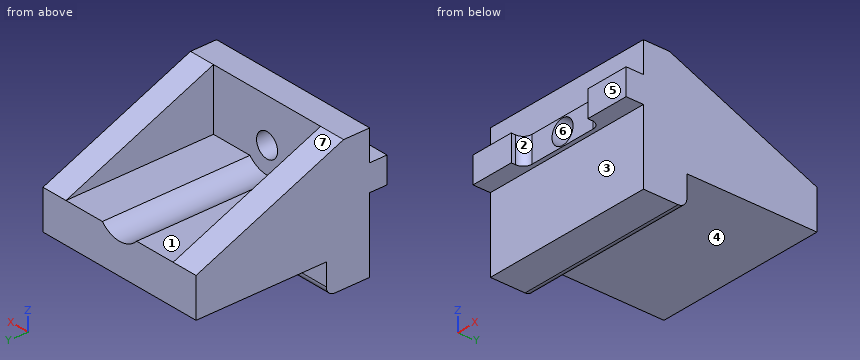
```python
from build123d import *

# Parameters (mm, degrees)
CROQUIS1_W              = 40
CROQUIS1_H              = 40
SALIENTE_EXTRUIR1_DEPTH = 20
CROQUIS2_W              = 28
CROQUIS2_H              = 14
CORTAR_EXTRUIR1_DEPTH   = 34
CORTAR_EXTRUIR2_DEPTH   = 40
CROQUIS7_W              = 40
CROQUIS7_H              = 6
SALIENTE_EXTRUIR2_DEPTH = 1
CROQUIS8_R              = 2.75
CORTAR_EXTRUIR6_DEPTH   = 7
CROQUIS9_R              = 6
CORTAR_EXTRUIR7_DEPTH   = 34
CROQUIS10_W             = 10
CROQUIS10_H             = 6
SALIENTE_EXTRUIR3_DEPTH = 3
REDONDEO1_R             = 2
SALIENTE_EXTRUIR5_DEPTH = 40
REDONDEO2_R             = 2


with BuildPart() as part:
    # Croquis1 → Saliente-Extruir1 (new body)
    with BuildSketch(Plane.XY):
        with Locations((20, -20)):
            Rectangle(CROQUIS1_W, CROQUIS1_H)
    extrude(amount=SALIENTE_EXTRUIR1_DEPTH)

    # Croquis2 → Cortar-Extruir1 (cut)
    with BuildSketch(Plane(origin=(0, 0, 0), x_dir=(1, 0, 0), z_dir=(0, 1, 0))):
        with Locations((20, -13)):
            Rectangle(CROQUIS2_W, CROQUIS2_H)
    extrude(amount=-CORTAR_EXTRUIR1_DEPTH, mode=Mode.SUBTRACT)

    # Croquis3 → Cortar-Extruir2 (cut)
    with BuildSketch(Plane.ZY):
        Polygon((20, 0), (20, -34), (6, 0), align=None)
    extrude(amount=-CORTAR_EXTRUIR2_DEPTH, mode=Mode.SUBTRACT)

    # Croquis7 → Saliente-Extruir2 (add)
    with BuildSketch(Plane.XZ.offset(40)):
        with Locations((20, 10)):
            Rectangle(CROQUIS7_W, CROQUIS7_H)
    extrude(amount=SALIENTE_EXTRUIR2_DEPTH)

    # Croquis8 → Cortar-Extruir6 (cut)
    with BuildSketch(Plane.XZ.offset(41)):
        with Locations((20, 10)):
            Circle(CROQUIS8_R)
    extrude(amount=-CORTAR_EXTRUIR6_DEPTH, mode=Mode.SUBTRACT)

    # Croquis9 → Cortar-Extruir7 (cut)
    with BuildSketch(Plane(origin=(0, -34, 0), x_dir=(1, 0, 0), z_dir=(0, 1, 0))):
        with Locations((20, -10)):
            Circle(CROQUIS9_R)
    extrude(amount=CORTAR_EXTRUIR7_DEPTH, mode=Mode.SUBTRACT)

    # Croquis10 → Saliente-Extruir3 (add)
    with BuildSketch(Plane.XZ.offset(41)):
        with Locations((5, 10)):
            Rectangle(CROQUIS10_W, CROQUIS10_H)
        with Locations((35, 10)):
            Rectangle(CROQUIS10_W, CROQUIS10_H)
    extrude(amount=SALIENTE_EXTRUIR3_DEPTH)

    # Redondeo1
    redondeo1_edges = [part.edges().sort_by_distance(p)[0] for p in [
        (10, -41, 10),
        (30, -41, 10),
    ]]
    fillet(redondeo1_edges, radius=REDONDEO1_R)

    # Croquis12 → Saliente-Extruir5 (add)
    with BuildSketch(Plane.ZY):
        Polygon((0, -40), (-10, -40), (-10, -30), (-3, -30), (-3, 0), (0, 0), align=None)
    extrude(amount=-SALIENTE_EXTRUIR5_DEPTH)

    # Redondeo2
    redondeo2_edges = [part.edges().sort_by_distance(p)[0] for p in [
        (20, -30, -10),
    ]]
    fillet(redondeo2_edges, radius=REDONDEO2_R)


solid = part.part
```
Can you work these out from the model? Positions are in its coordinate system, mm. Face numbers are marked on the shaded views. A direction names the side the tool comes from. Coordinates: 2 decimals unless noted, no trailing zeros. Loops run counter-clockwise (first coordinate to the right, second up) from the corner with the lowest first, then second, coordinate; pieces in that order, holes last. Notation, with made-up numbers: (63.5, -19.5) - (68.5, -19.5) arc R27 cw to (68.5, 4.5) - close; hole circle Ø8 at (65.5, 89.25). An arc over 180 degrees is marked (long way). Answer as CSV lines item,"result". Start each with the question number.
1) Suppose I cut it at A-A (x = 20). Please give me the cut outline in (y, z), plus the area to 3 significant figures.
2) Which directions (+Z, -Z, +X, -X, +Y, -Y) give clear straight access to the entire face, cutting with the end or side of a thin tool? Please do the marked faces 1, 2 and 3.
3) Suppose I cut it at D-D (x = 36). Please give me the cut outline in (y, z), plus the area to 3 significant figures.
4) For pin 1 (1.5 mm diameter, centred on x = 11, z = -5, fed in from +Y); pin 2 (5 mm diameter, centred on x = 25.5, z = 14, fed in from +Y); pin 3 (1 mm diameter, centred on x = 32.5, y = -25.5, fed in from +Z), each with a flat end and sliding along its axis, tell me the tip position at first contact or that it passes through.
5) Thinking about a two-plate mould opening in Z: for the marked faces 4, 5, 6 and 7, which applies, pulls with the +Z half, pulls with the -Z half, needs draft (parallel to the pull), parting line crosses it, or undercut?
6) I need wall thicknesses on line 1 (Z direction, x = 20, y = -39.5); line 2 (X direction, y = -20, z = 7.75); line 3 (Z direction, x = 27, y = -13). Which ranges of each line are inside material? Lowest first, please. Write a range as from..to.
7) Suppose I cut it at B-B (y = -38). Please give me the cut outline in (x, z), plus the area to 3 significant figures.
8) Suppose I cut it at C-C (z = 10). Please give me the cut outline in (x, y), plus the area to 3 significant figures.
Check result:
1,outline,"(-41, 7) - (-40, 7) - (-40, -10) - (-32, -10) arc R2 ccw to (-30, -8) - (-30, -3) - (0, -3) - (0, 4) - (-34, 4) - (-34, 7.25) - (-41, 7.25) - close; (-41, 12.75) - (-34, 12.75) - (-34, 20) - (-40, 20) - (-40, 13) - (-41, 13) - close"
1,area,"413 mm²"
2,face 1,"+Z, +Y"
2,face 2,"+Z, -Z, -Y"
2,face 3,"-Z, +X, -X, -Y"
3,outline,"(-44, 7) - (-40, 7) - (-40, -10) - (-32, -10) arc R2 ccw to (-30, -8) - (-30, -3) - (0, -3) - (0, 6) - (-34, 20) - (-40, 20) - (-40, 13) - (-44, 13) - close"
3,area,"775 mm²"
4,pin 1,"stops at y = -30"
4,pin 2,"stops at y = -34"
4,pin 3,"stops at z = 6"
5,face 4,"pulls with the -Z half"
5,face 5,"needs draft"
5,face 6,"undercut"
5,face 7,"pulls with the +Z half"
6,line 1,"z = -10..7.25, 12.75..20"
6,line 2,"x = 0..6, 34..40"
6,line 3,"z = -3..6"
7,outline,"(0, -10) - (40, -10) - (40, 20) - (0, 20) - close; hole circle Ø5.5 at (20, 10)"
7,area,"1,180 mm²"
8,outline,"(0, -44) - (10, -44) - (10, -43) arc R2 cw to (12, -41) - (17.25, -41) - (17.25, -34) - (6, -34) - (6, -9.71) - (0, -9.71) - close; (22.75, -41) - (28, -41) arc R2 cw to (30, -43) - (30, -44) - (40, -44) - (40, -9.71) - (34, -9.71) - (34, -34) - (22.75, -34) - close"
8,area,"595 mm²"
